from build123d import *

# Parameters (mm, degrees)
F0_W      = 23.7236
F0_H      = 15.7734
F2_DEPTH  = 9.6012
F1_R      = 2.4511
F3_DEPTH  = 1.9812
F4_W      = 21.2344
F4_H      = 13.2842
F6_DEPTH  = 7.62
F5_R      = 3.2258
F7_DEPTH  = 8.89
F8_R      = 2.467308
F9_R      = 2.45607
F10_DEPTH = 7.62


with BuildPart() as f2:
    # F0 (on Top) → F2 (new body)
    with BuildSketch(Plane.XY):
        Rectangle(F0_W, F0_H)
    extrude(amount=-F2_DEPTH)

    # F1 (on face) → F3 (join)
    with BuildSketch(Plane.XY):
        with Locations((-7.9756, 3.9624)):
            Circle(F1_R)
        with Locations((0, 3.9624)):
            Circle(F1_R)
        with Locations((7.9756, 3.9624)):
            Circle(F1_R)
        with Locations((7.9756, -3.9624)):
            Circle(F1_R)
        with Locations((0, -3.9624)):
            Circle(F1_R)
        with Locations((-7.9756, -3.9624)):
            Circle(F1_R)
    extrude(amount=F3_DEPTH)

    # F4 (on face) → F6 (cut)
    with BuildSketch(Plane(origin=(0, 0, -9.6012), x_dir=(1, 0, 0), z_dir=(0, 0, -1))):
        Rectangle(F4_W, F4_H)
    extrude(amount=-F6_DEPTH, mode=Mode.SUBTRACT)

    # F5 (on face) → F7 (join)
    with BuildSketch(Plane(origin=(0, 0, -9.6012), x_dir=(1, 0, 0), z_dir=(0, 0, -1))):
        with Locations((-3.556, 0)):
            Circle(F5_R)
        with Locations((3.556, 0)):
            Circle(F5_R)
    extrude(amount=-F7_DEPTH)

    # F8 (on face) + F9 (on face) → F10 (cut)
    with BuildSketch(Plane(origin=(0, 0, -9.6012), x_dir=(1, 0, 0), z_dir=(0, 0, -1))):
        with Locations((-3.556, 0)):
            Circle(F8_R)
    with BuildSketch(Plane(origin=(0, 0, -9.6012), x_dir=(1, 0, 0), z_dir=(0, 0, -1))):
        with Locations((3.556, 0)):
            Circle(F9_R)
    extrude(amount=-F10_DEPTH, mode=Mode.SUBTRACT)


solid = f2.part
The listing builds one solid part. Answer for the finished solid, in the listing's coordinates (mm). A direction names the side the tool comes from. Round coordinates to 2 decimals unless told otherwise and drop trailing zeros. Order: outer loops, then holes, each group sorted by start corner. A loop starts at its lowest first (then second) coordinate and runs counter-clockwise, first axis right, second up. Notation, with made-up numbers: (-32.5, -5.5) - (18.5, -5.5) arc R36 cw to (18.5, 31.5) - close; hole circle Ø4 at (66.25, -5.75). An arc over 180 degrees is marked (long way). Write item = value, one per line. Start each with the question number.
1) Section D-D, the plane y = -4.5 is taken. Write down the section's boundary in (x, z).
2) Straight lines are drawn through the part: L1, parallel to X at y = 0, z = -7; L2, parallel to Y at x = 9.5, z = -5.75; L3, parallel to X at y = 5, z = -9. For each, find the intervals that lie inside material, in ascending order.
3) Section A-A, the plane z = -6.5 is taken. Write down the section's boundary in (x, y), plus the area to 3 significant figures.
4) For faces 4 (the cylindrical face through (6.633, -0.969, -5.845)), 5 (the flat face through (-8, -4, 1.981)), 6 (the cylindrical face through (-6.658, -1.896, 0.977)), determine the directions among +Z, -Z, +X, -X, +Y, -Y from which every point of the face is accessible in a straight line to the end or side of a thin tool.
5) Given pin 1 (3 mm diameter, centred on x = 3.556, y = 0, fed in from +Z), flat-ended and moving along its own axis, determine where the tip first touches the part or whether it passes through.
6) Section B-B, the plane x = 0 is taken. Write down the section's boundary in (y, z), plus the area to 3 significant figures.
7) Section C-C, the plane y = 0 is taken. Write down the section's boundary in (x, z), plus the area to 3 significant figures.
8) For a pull along Y with two mould halves and no side action, classify faces 1 (the flat face through (8, 4, 1.981)), 2 (the flat face through (0, -7.887, -5)), 3 (the flat face through (0, -6.642, -6)) as released by +Y, released by -Y, zero draft, split by the parting line, or undercut.
Results list:
q1.outline = (-11.86, -9.6) - (-10.62, -9.6) - (-10.62, -1.98) - (10.62, -1.98) - (10.62, -9.6) - (11.86, -9.6) - (11.86, 0) - (10.37, 0) - (10.37, 1.98) - (5.58, 1.98) - (5.58, 0) - (2.39, 0) - (2.39, 1.98) - (-2.39, 1.98) - (-2.39, 0) - (-5.58, 0) - (-5.58, 1.98) - (-10.37, 1.98) - (-10.37, 0) - (-11.86, 0) - close
q2.L1 = -11.86 to -10.62, -6.78 to -6.02, -1.09 to -0.33, 0.33 to 1.1, 6.01 to 6.78, 10.62 to 11.86
q2.L2 = -7.89 to -6.64, 6.64 to 7.89
q2.L3 = -11.86 to -10.62, 10.62 to 11.86
q3.outline = (-11.86, -7.89) - (11.86, -7.89) - (11.86, 7.89) - (-11.86, 7.89) - close; circle Ø6.45 at (-3.56, 0); circle Ø6.45 at (3.56, 0); hole (-10.62, -6.64) - (10.62, -6.64) - (10.62, 6.64) - (-10.62, 6.64) - close; hole circle Ø4.93 at (-3.56, 0); hole circle Ø4.91 at (3.56, 0)
q3.area = 119 mm^2
q4.face_4 = -Z
q4.face_5 = +Z, +X, -X, +Y, -Y
q4.face_6 = +Z
q5.pin_1 = 0
q6.outline = (-7.89, -9.6) - (-6.64, -9.6) - (-6.64, -1.98) - (6.64, -1.98) - (6.64, -9.6) - (7.89, -9.6) - (7.89, 0) - (6.41, 0) - (6.41, 1.98) - (1.51, 1.98) - (1.51, 0) - (-1.51, 0) - (-1.51, 1.98) - (-6.41, 1.98) - (-6.41, 0) - (-7.89, 0) - close
q6.area = 69.6 mm^2
q7.outline = (-11.86, -9.6) - (-10.62, -9.6) - (-10.62, -1.98) - (-6.78, -1.98) - (-6.78, -9.6) - (-6.02, -9.6) - (-6.02, -1.98) - (-1.09, -1.98) - (-1.09, -9.6) - (-0.33, -9.6) - (-0.33, -1.98) - (0.33, -1.98) - (0.33, -9.6) - (1.1, -9.6) - (1.1, -1.98) - (6.01, -1.98) - (6.01, -9.6) - (6.78, -9.6) - (6.78, -1.98) - (10.62, -1.98) - (10.62, -9.6) - (11.86, -9.6) - (11.86, 0) - (-11.86, 0) - close
q7.area = 89.3 mm^2
q8.face_1 = zero draft
q8.face_2 = released by -Y
q8.face_3 = undercut
